Could you check a few things on this model? Use its own coordinates, in mm. A direction names the side the tool comes from. Round coordinates to 2 decimals unless told otherwise and drop trailing zeros. Loops run counter-clockwise (first coordinate to the right, second up) from the corner with the lowest first, then second, coordinate; pieces in that order, holes last. Notation, with made-up numbers: (-20.5, -9) -> (15.5, -9) arc R19 ccw to (15.5, 20) -> close; hole circle Ø10 at (-30.5, 73). An arc over 180 degrees is marked (long way). Use CSV: the item, a comma, the result in double quotes. Start each with the question number.
```python
from build123d import *

# Parameters (mm, degrees)
BOSS_EXTRUDE1_DEPTH  = 6.35
CAVITY1_START        = 298.45
CAVITY1_OUTLINE_R    = 12.7
CAVITY1_DEPTH        = 12.7
CAVITY1_START_2      = 720.91620239
CAVITY1_2_DEPTH      = 22.43918751
SKETCH2_W            = 22.270177668
SKETCH2_H            = 113.672619585
CUT_EXTRUDE1_DEPTH   = 1143.349273427
MOVE_FACE_SLOTS_BY   = 0.762
MOVE_FACE_SLOTS_2_BY = 0.762
MOVE_FACE_SLOTS_3_BY = 0.762
MOVE_FACE_SLOTS_4_BY = 0.762
MOVE_FACE_SLOTS_5_BY = 0.762
MOVE_FACE_SLOTS_6_BY = 0.762
MOVE_FACE_HOLE_BY    = 0.635
SLOT_FILLET_R        = 3.175


# Read off the part's stored shape, not the designer's step: Cavity1
with BuildPart() as part:
    # Sketch1 → Boss-Extrude1 (new, symmetric)
    with BuildSketch(Plane(origin=(0, 304.8, 0), x_dir=(1, 0, 0), z_dir=(0, 1, 0))):
        Polygon((798.4, -133.35), (1001.6, -133.35), (1001.6, -260.35), (1014.3, -260.35), (1014.3, -133.35), (1065.1, -133.35), (1065.1, -412.75), (1014.3, -412.75), (1001.6, -412.75), (798.4, -412.75), (785.7, -412.75), (734.9, -412.75), (734.9, -133.35), (785.7, -133.35), (785.7, -260.35), (798.4, -260.35), align=None)
    extrude(amount=BOSS_EXTRUDE1_DEPTH, both=True)

    # Cavity1 outline → Cavity1 (cut)
    with BuildSketch(Plane(origin=(0, 0, 0), x_dir=(1, 0, 0), z_dir=(0, 1, 0)).offset(CAVITY1_START)):
        with Locations((900, -250)):
            Circle(CAVITY1_OUTLINE_R)
    extrude(amount=CAVITY1_DEPTH, mode=Mode.SUBTRACT)

    # Cavity1 2 outline → Cavity1 2 (cut)
    with BuildSketch(Plane(origin=(0, 0, 0), x_dir=(0.7149295353100829, -0.698752516444498, 0.02491345627949748), z_dir=(0.6991965099607612, 0.7144755512387372, -0.025474048378572107)).offset(CAVITY1_START_2)):
        with BuildLine():
            Line((312, -255.374549574), (314.076314529, -255.435688643))
            ThreePointArc((314.076314529, -255.435688643), (327.146171675, -242.424687318), (313.444242413, -230.081087528))
            Line((313.444242413, -230.081087528), (312, -230.195835843))
            Line((312, -230.195835843), (312, -255.374549574))
        make_face()
    extrude(amount=CAVITY1_2_DEPTH, mode=Mode.SUBTRACT)

    # Sketch2 → Cut-Extrude1 (cut, through all)
    with BuildSketch(Plane(origin=(0, 311.15, 0), x_dir=(1, 0, 0), z_dir=(0, 1, 0))):
        with Locations((746.035088834, -190.186309793)):
            Rectangle(SKETCH2_W, SKETCH2_H)
    extrude(amount=-CUT_EXTRUDE1_DEPTH, mode=Mode.SUBTRACT)

    # Move Face Slots: a face moved inward by 0.762
    extrude(part.faces().sort_by_distance((1014.3, 304.8, 196.85))[0], amount=MOVE_FACE_SLOTS_BY, dir=(1, 0, 0), mode=Mode.SUBTRACT)

    # Move Face Slots 2: a face moved inward by 0.762
    extrude(part.faces().sort_by_distance((1007.95, 304.8, 260.35))[0], amount=MOVE_FACE_SLOTS_2_BY, dir=(0, 0, 1), mode=Mode.SUBTRACT)

    # Move Face Slots 3: a face moved inward by 0.762
    extrude(part.faces().sort_by_distance((1001.6, 304.8, 196.85))[0], amount=MOVE_FACE_SLOTS_3_BY, dir=(-1, 0, 0), mode=Mode.SUBTRACT)

    # Move Face Slots 4: a face moved inward by 0.762
    extrude(part.faces().sort_by_distance((785.7, 304.8, 196.85))[0], amount=MOVE_FACE_SLOTS_4_BY, dir=(-1, 0, 0), mode=Mode.SUBTRACT)

    # Move Face Slots 5: a face moved inward by 0.762
    extrude(part.faces().sort_by_distance((792.05, 304.8, 260.35))[0], amount=MOVE_FACE_SLOTS_5_BY, dir=(0, 0, 1), mode=Mode.SUBTRACT)

    # Move Face Slots 6: a face moved inward by 0.762
    extrude(part.faces().sort_by_distance((798.4, 304.8, 196.85))[0], amount=MOVE_FACE_SLOTS_6_BY, dir=(1, 0, 0), mode=Mode.SUBTRACT)

    # Move Face Hole: a curved face moved inward by 0.635
    add(Solid.thicken(part.faces().sort_by_distance((887.3, 304.8, 250))[0], -MOVE_FACE_HOLE_BY), mode=Mode.SUBTRACT)

    # Slot Fillet
    slot_fillet_edges = [part.edges().sort_by_distance(p)[0] for p in [
        (1015.062, 304.8, 133.35),
        (1015.062, 304.8, 261.112),
        (1000.838, 304.8, 261.112),
        (1000.838, 304.8, 133.35),
        (799.162, 304.8, 133.35),
        (799.162, 304.8, 261.112),
        (784.938, 304.8, 261.112),
        (784.938, 304.8, 133.35),
    ]]
    fillet(slot_fillet_edges, radius=SLOT_FILLET_R)


solid = part.part
```
1. Suppose I cut it at A-A (x = 900). List the corners of the cut face in (y, z) for me (3 decimals), then the cut area to 3 significant figures.
2. Suppose I cut it at C-C (y = 303.5). List the corners of the cut face in (x, z) for me (3 decimals).
3. Will these pins go through, and if not, where does the flat tip stop? pin 1 (6.5 mm diameter, centred on y = 302, z = 220, fed in from -X); pin 2 (4 mm diameter, centred on x = 792, y = 302, fed in from -Z).
4. If I drill on L1, parallel to X at y = 306, z = 250 (3 decimals); L2, parallel to X at y = 308, z = 171; L3, parallel to Z at x = 900, y = 305.5 (3 decimals), over which ranges is the centre line in solid material (lowest first)?
5. We'd pull the mould along Z, two halves only. Please class faces 1 (the face through (886.68, 304.71, 249.41)), 2 (the face through (1008, 305, 261.112)), 3 (the face through (1015.062, 305, 198)): pulls with the +Z half, pulls with the -Z half, needs draft (parallel to the pull), parting line crosses it, or undercut.
6. For faces 4 (the face through (784.938, 305, 196)), 5 (the face through (899, 305, 133.35)), 6 (the face through (746, 305, 247.023)), which set-ups out of +Z, -Z, +X, -X, +Y, -Y let a thin tool reach every point of the face, with its end or its side?
7. Suppose I cut it at B-B (z = 213). List the corners of the cut face in (x, y) for me.
Geometry check:
1,outline,"(298.45, 133.35) -> (311.15, 133.35) -> (311.15, 236.665) -> (298.45, 236.665) -> close; (298.45, 263.335) -> (311.15, 263.335) -> (311.15, 412.75) -> (298.45, 412.75) -> close"
1,area,"3,210 mm²"
2,outline,"(734.9, 247.023) -> (757.17, 247.023) -> (757.17, 133.35) -> (781.763, 133.35) arc R3.175 ccw to (784.938, 136.525) -> (784.938, 257.937) arc R3.175 cw to (788.113, 261.112) -> (795.987, 261.112) arc R3.175 cw to (799.162, 257.937) -> (799.162, 136.525) arc R3.175 ccw to (802.337, 133.35) -> (997.663, 133.35) arc R3.175 ccw to (1000.838, 136.525) -> (1000.838, 257.937) arc R3.175 cw to (1004.013, 261.112) -> (1011.887, 261.112) arc R3.175 cw to (1015.062, 257.937) -> (1015.062, 136.525) arc R3.175 ccw to (1018.237, 133.35) -> (1065.1, 133.35) -> (1065.1, 412.75) -> (734.9, 412.75) -> close; hole circle Ø26.67 at (900, 250)"
3,pin 1,"stops at x = 757.17"
3,pin 2,"stops at z = 261.11"
4,L1,"x = 734.9 to 784.938, 799.162 to 886.665, 913.335 to 1000.838, 1015.062 to 1065.1"
4,L2,"x = 757.17 to 784.94, 799.16 to 1000.84, 1015.06 to 1065.1"
4,L3,"z = 133.35 to 236.665, 263.335 to 412.75"
5,face 1,"undercut"
5,face 2,"pulls with the -Z half"
5,face 3,"needs draft"
6,face 4,"-Z, +Y, -Y"
6,face 5,"-Z, +X, -X, +Y, -Y"
6,face 6,"-Z, -X, +Y, -Y"
7,outline,"(757.17, 298.45) -> (784.94, 298.45) -> (784.94, 311.15) -> (757.17, 311.15) -> close; (799.16, 298.45) -> (1000.84, 298.45) -> (1000.84, 311.15) -> (799.16, 311.15) -> close; (1015.06, 298.45) -> (1065.1, 298.45) -> (1065.1, 311.15) -> (1015.06, 311.15) -> close"
